Autodesk Inventor part; units mm, degrees
ref_plane "MidSidePlane" through (0, 0, 10) normal (0, 0, 1) x (1, 0, 0)
ref_plane "YZ Plane" through (0, 0, 0) normal (1, 0, 0) x (0, 1, 0)
ref_plane "XZ Plane" through (0, 0, 0) normal (0, 1, 0) x (-1, 0, 0)
sketch "ShaftProfile" plane through (0, 0, 0) normal (0, 0, 1) x (1, 0, 0)
  line L0 (-53, 0) -> (52, 0) construction
  line L1 (-38, 9) -> (37, 9)
  line L2 (37, 9) -> (37, 0)
  line L3 (-38, 0) -> (-38, 9)
  line L4 (-38, 0) -> (37, 0)
  point P0 (0, 0)
  dimension "d1" = 75
  dimension "d2" = 9
  dimension "d4" = 38
revolve "ShaftFeature" add sketch "ShaftProfile" angle 360 about axis through (-38, 0, 0) along (1, 0, 0)
sketch "Sketch2" plane through (-38, 0, 0) normal (-1, 0, 0) x (0, 0, 1)
  circle A0 centre (0, 0) radius 9
hole "ShaftHoleFeature" at (-38, 0, 0) direction (1, 0, 0) diameter 16 end through all
ref_plane "MidSidePlane" through (0, 0, 10) normal (0, 0, 1) x (1, 0, 0)
sketch "CapHoles" plane through (0, 0, 10) normal (0, 0, 1) x (1, 0, 0)
  line L0 (37, -9) -> (37, 9) construction
  line L1 (-38, -9) -> (-38, 9) construction
  line L2 (-57, 0) -> (76, 0) construction
  circle A0 centre (-33.5, 0) radius 1.25
  circle A1 centre (32.5, 0) radius 1.25
  dimension "d24" = 2.5
  dimension "d25" = 4.5
  dimension "d26" = 4.5
extrude "CapHolesFeature" cut sketch "CapHoles" against normal through all
equation "\"d26\" = d25"
properties part number "BackPair1PistonShaft"
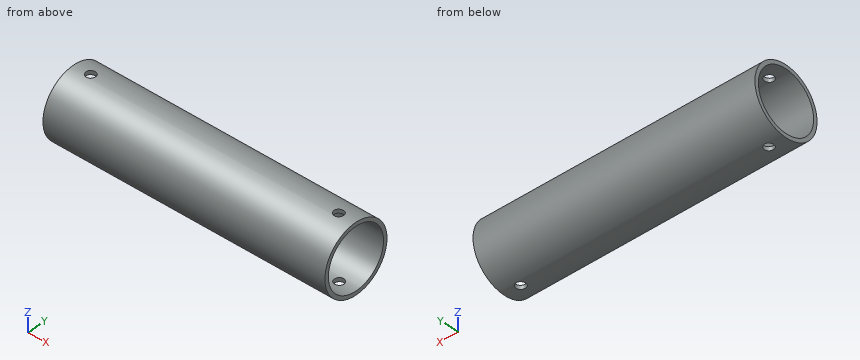
Here's how the part is built. I have some questions about the finished solid (model axes, mm). Coordinates: 2 decimals unless noted, no trailing zeros. Write each loop counter-clockwise with the first axis right and the second up, starting at its lowest first coordinate (ties: lowest second). Pieces come first, ordered by that corner, then holes. Notation, with made-up numbers: M -24.75,83 L -18.75,83 A28 ccw -18.75,107 Z; hole C 6,60.25 d9. An arc over 180 degrees is marked long. Answer as CSV lines item,"result". Start each with the question number.
Q1. I need wall thicknesses on probe 1 along X at (y, z) = (0, -8.45); probe 2 along Z at (x, y) = (31, 0); probe 3 along Y at (x, z) = (-4, -2.25). Which ranges of each line are inside material? Lowest first, please. Write a range as [from, to].
Q2. Suppose I cut it at B-B, the plane y = 0. List the corners of the cut face in (x, z) for me, then the cut area to 3 significant figures.
Q3. Suppose I cut it at D-D, the plane x = -8.5. List the corners of the cut face in (y, z) for me.
Q4. Will these pins go through, and if not, where does the flat tip stop? pin 1 Ø3 at (x, z) = (20.5, -7) entering from +Y; pin 2 Ø3 at (y, z) = (2, 7) entering from +X; pin 3 Ø8 at (x, y) = (-18.5, 6.5) entering from +Z; pin 4 Ø1 at (x, y) = (-16, 5.5) entering from +Z.
Q5. Suppose I cut it at A-A, the plane z = 0. List the corners of the cut face in (x, y) for me, then the cut area to 3 significant figures.
Q6. Suppose I cut it at C-C, the plane x = -33.5. List the corners of the cut face in (y, z) for me, then the cut area to 3 significant figures.
Entries:
1,probe 1,"x = [-38, -34.75], [-32.25, 31.25], [33.75, 37]"
1,probe 2,"z = [-9, -8], [8, 9]"
1,probe 3,"y = [-8.71, -7.68], [7.68, 8.71]"
2,outline,"M -38,-9 L -34.75,-9 L -34.75,-8 L -38,-8 Z; M -38,8 L -34.75,8 L -34.75,9 L -38,9 Z; M -32.25,-9 L 31.25,-9 L 31.25,-8 L -32.25,-8 Z; M -32.25,8 L 31.25,8 L 31.25,9 L -32.25,9 Z; M 33.75,-9 L 37,-9 L 37,-8 L 33.75,-8 Z; M 33.75,8 L 37,8 L 37,9 L 33.75,9 Z"
2,area,"140 mm²"
3,outline,"C 0,0 d18; hole C 0,0 d16"
4,pin 1,"stops at y = 7.12"
4,pin 2,"stops at x = 37"
4,pin 3,"stops at z = 8.65"
4,pin 4,"stops at z = 7.48"
5,outline,"M -38,-9 L 37,-9 L 37,-8 L -38,-8 Z; M -38,8 L 37,8 L 37,9 L -38,9 Z"
5,area,"150 mm²"
6,outline,"M -1.25,-8.91 L -1.25,-7.9 A8 cw -1.25,7.9 L -1.25,8.91 A9 ccw Z; M 1.25,-8.91 A9 ccw 1.25,8.91 L 1.25,7.9 A8 cw 1.25,-7.9 Z"
6,area,"48.4 mm²"
